Autodesk Inventor part; units mm, degrees
ref_plane "Work Plane1" through (0, -11.5, 75) normal (0, 0, 1) x (1, 0, 0)
ref_plane "YZ Plane" through (0, 0, 0) normal (1, 0, 0) x (0, 1, 0)
ref_plane "XZ Plane" through (0, 0, 0) normal (0, 1, 0) x (-1, 0, 0)
sketch "Sketch1" plane through (0, 0, 0) normal (1, 0, 0) x (0, 1, 0)
  line L0 (0, 0) -> (4.5, 0)
  line L1 (4.5, 0) -> (4.5, 43)
  line L2 (4.5, 43) -> (0, 43)
  line L3 (0, 43) -> (0, 0)
  line L4 (4.5, 43) -> (8.9259, 26.4824)
  line L5 (4.5, 21.5) -> (10.3528, 21.5)
  line L6 (13, 25) -> (10.8577, 25)
  line L7 (25.5, 39.5) -> (30, 39.5)
  line L8 (30, 39.5) -> (30, 3.5)
  line L9 (30, 3.5) -> (25.5, 3.5)
  line L10 (25.5, 3.5) -> (25.5, 39.5)
  line L11 (25.5, 39.5) -> (22.0119, 26.4824)
  line L12 (10.8577, 18) -> (20.0801, 18)
  line L13 (4.5, 0) -> (8.9259, 16.5176)
  line L14 (25.5, 3.5) -> (22.0119, 16.5176)
  line L15 (3, 25) -> (20.0801, 25)
  arc A0 (8.9259, 26.4824) -> (10.8577, 25) centre (10.8577, 27) ccw
  arc A1 (20.0801, 25) -> (22.0119, 26.4824) centre (20.0801, 27) ccw
  arc A2 (22.0119, 16.5176) -> (20.0801, 18) centre (20.0801, 16) ccw
  arc A3 (10.8577, 18) -> (8.9259, 16.5176) centre (10.8577, 16) ccw
  line L16 (-11.5, 16.5176) -> (-11.5, 3.5)
  point P0 (9.6974, 23.6032)
  point P1 (21.6069, 24.9709)
  point P2 (3, 18)
  point P3 (23.25, 18)
  point P4 (9.6974, 19.3968)
  point P5 (21.6069, 18.0291)
  point P6 (23.25, 25)
  dimension "d0" = 43
  dimension "d1" = 4.5
  dimension "d2" = 15
  dimension "d3" = 21.5
  dimension "d4" = 3.5
  dimension "d5" = 4.5
  dimension "d6" = 36
  dimension "d7" = 18
  dimension "d8" = 15
  dimension "d9" = 3.5
  dimension "d10" = 30
  dimension "d11" = 2
  dimension "d12" = 32
revolve "Revolution1" add sketch "Sketch1" angle 360 about axis through (0, -11.5, 16.5176) along (0, 0, -1)
ref_plane "Work Plane1" through (0, -11.5, 75) normal (0, 0, 1) x (1, 0, 0)
sketch "Sketch2" plane through (0, -11.5, 75) normal (0, 0, 1) x (1, 0, 0)
  line L0 (9.2559, 22.3457) -> (12.1824, 29.4109)
  line L1 (22.3457, 9.2559) -> (27.1721, 11.2551)
  line L2 (0, 0) -> (0, 29.4109)
  line L3 (0, 0) -> (29.4109, 0)
  arc A0 (27.3903, 11.3454) -> (11.3454, 27.3903) centre (0, 0) ccw
  line L4 (22.3457, 9.2559) -> (27.1721, 11.2551)
  line L5 (22.3457, 9.2559) -> (27.3903, 11.3454)
  line L6 (22.3457, 9.2559) -> (27.3903, 11.3454)
  arc A1 (22.3457, 9.2559) -> (9.2559, 22.3457) centre (0, 0) ccw
  arc A2 (0, 24.1868) -> (24.1868, 0) centre (0, 0) ccw
  line L7 (11.3454, 27.3903) -> (9.2559, 22.3457)
  line L8 (27.3903, 11.3454) -> (22.3457, 9.2559)
  arc A3 (22.3457, 9.2559) -> (9.2559, 22.3457) centre (0, 0) ccw
  arc A4 (27.3903, 11.3454) -> (11.3454, 27.3903) centre (0, 0) ccw
  line L9 (9.2559, -22.3457) -> (12.1824, -29.4109)
  line L10 (22.3457, -9.2559) -> (27.1721, -11.2551)
  arc A5 (11.3454, -27.3903) -> (27.3903, -11.3454) centre (0, 0) ccw
  line L11 (22.3457, -9.2559) -> (27.1721, -11.2551)
  line L12 (22.3457, -9.2559) -> (27.3903, -11.3454)
  line L13 (22.3457, -9.2559) -> (27.3903, -11.3454)
  arc A6 (9.2559, -22.3457) -> (22.3457, -9.2559) centre (0, 0) ccw
  line L14 (11.3454, -27.3903) -> (9.2559, -22.3457)
  line L15 (27.3903, -11.3454) -> (22.3457, -9.2559)
  arc A7 (9.2559, -22.3457) -> (22.3457, -9.2559) centre (0, 0) ccw
  arc A8 (11.3454, -27.3903) -> (27.3903, -11.3454) centre (0, 0) ccw
  line L16 (0, 0) -> (0, -24.1868)
  line L17 (-9.2559, 22.3457) -> (-12.1824, 29.4109)
  line L18 (-22.3457, 9.2559) -> (-27.1721, 11.2551)
  arc A9 (-11.3454, 27.3903) -> (-27.3903, 11.3454) centre (0, 0) ccw
  line L19 (-22.3457, 9.2559) -> (-27.1721, 11.2551)
  line L20 (-22.3457, 9.2559) -> (-27.3903, 11.3454)
  line L21 (-22.3457, 9.2559) -> (-27.3903, 11.3454)
  arc A10 (-9.2559, 22.3457) -> (-22.3457, 9.2559) centre (0, 0) ccw
  line L22 (-11.3454, 27.3903) -> (-9.2559, 22.3457)
  line L23 (-27.3903, 11.3454) -> (-22.3457, 9.2559)
  arc A11 (-9.2559, 22.3457) -> (-22.3457, 9.2559) centre (0, 0) ccw
  arc A12 (-11.3454, 27.3903) -> (-27.3903, 11.3454) centre (0, 0) ccw
  line L24 (-22.3457, -9.2559) -> (-27.1721, -11.2551)
  line L25 (-22.3457, -9.2559) -> (-27.1721, -11.2551)
  line L26 (-22.3457, -9.2559) -> (-27.3903, -11.3454)
  line L27 (-22.3457, -9.2559) -> (-27.3903, -11.3454)
  line L28 (-27.3903, -11.3454) -> (-22.3457, -9.2559)
  arc A13 (-22.3457, -9.2559) -> (-9.2559, -22.3457) centre (0, 0) ccw
  arc A14 (-22.3457, -9.2559) -> (-9.2559, -22.3457) centre (0, 0) ccw
  arc A15 (-27.3903, -11.3454) -> (-11.3454, -27.3903) centre (0, 0) ccw
  line L29 (-11.3454, -27.3903) -> (-9.2559, -22.3457)
  line L30 (-9.2559, -22.3457) -> (-12.1824, -29.4109)
  arc A16 (-27.3903, -11.3454) -> (-11.3454, -27.3903) centre (0, 0) ccw
  point P0 (0, 11.5)
  point P1 (-29.4109, 0)
  point P2 (-24.1868, 0)
  point P3 (-9.2559, 22.3457)
  point P4 (9.2559, -22.3457)
  point P5 (27.1721, -11.2551)
  point P6 (22.3457, -9.2559)
  point P7 (-22.3457, -9.2559)
  point P8 (-27.1721, -11.2551)
  dimension "d15" = 29.4109
  dimension "d16" = 22.5
  dimension "d17" = 22.5
extrude "Extrusion1" cut sketch "Sketch2" against normal through all contours L0 A0 L5 L1 A1 | A2 L18 L20 A9 L17 | L10 L12 A5 L9 A2 | L29 A15 L26 L24 A2
equation "\"d3\" = 0.5 * d0"
equation "\"d7\" = 0.5 * d6"
properties part number "roller"
Work out the finished part from the listing and answer in its coordinate system (mm). A direction names the side the tool comes from. Round coordinates to 2 decimals unless told otherwise and drop trailing zeros. Loops run counter-clockwise (first coordinate to the right, second up) from the corner with the lowest first, then second, coordinate; pieces in that order, holes last. Notation, with made-up numbers: (-34, 43) -> (-7, 43) arc R24 ccw to (-7, 77) -> close; hole circle Ø3 at (40, 48). An arc over 180 degrees is marked (long way). Write each question's results on one line, items separated by ' | '. Start each with the question number.
1. Section D-D (z = 33.5) is taken. Determine the outline of the cut face in (x, y).
2. Find the intervals of material crossed by probe 1 along X at (y, z) = (-11, 15); probe 2 along X at (y, z) = (-11.5, 12.5); probe 3 along Y at (x, z) = (24, 22.5), in increasing order. Write a range as from..to.
3. For a pull along Y with two mould halves and no side action, classify faces 1 (the face through (-25.252, -44.433, 21.248)), 2 (the face through (-7, -1, 43)), 3 (the face through (-10.315, -36.403, 21.549)) as +Y half, -Y half, draft (parallel to the pull), parting line (faces both ways), or undercut.
4. Given pin 1 Ø1 at (x, z) = (28, 23) entering from -Y; pin 2 Ø3 at (x, z) = (-3.5, 24.5) entering from -Y; pin 3 Ø10 at (y, z) = (-22.5, 23.5) entering from -X, each flat-ended and moving along its own axis, determine where each tip first touches the part or whether it passes through.
5. Section C-C (z = 21) is taken. Determine the outline of the cut face in (x, y).
6. A tool of negligible diameter and unlimited length cuts with its end or side. For faces 4 (the face through (17.008, -28.696, 21.549)), 5 (the face through (-21, -2, 18)), 6 (the face through (-21, -2, 25)), from which of +Z, -Z, +X, -X, +Y, -Y can it reach the whole face along a straight path? Write none if from no direction.
Evaluation:
1) outline: circle Ø83 at (0, -11.5); circle Ø37.09 at (0, -11.5); hole circle Ø70.78 at (0, -11.5); hole circle Ø23 at (0, -11.5)
2) probe 1: x = -41.5..-33.91, -20.01..-11.49, 11.49..20.01, 33.91..41.5 | probe 2: x = -41.5..-34.59, -19.35..-11.5, 11.5..19.35, 34.59..41.5 | probe 3: y = -45.36..-28.91, -21.44..-1.56, 5.91..22.36
3) face 1: parting line | face 2: draft | face 3: undercut
4) pin 1: stops at y = -42.58 | pin 2: stops at y = -52.95 | pin 3: stops at x = -41.06
5) outline: circle Ø83 at (0, -11.5); hole (-27.39, -22.85) arc R29.65 ccw to (-11.35, -38.89) -> (-9.26, -33.85) arc R24.19 cw to (-22.35, -20.76) -> (-27.17, -22.76) -> close; hole (-27.39, -0.15) -> (-27.17, -0.24) -> (-22.35, -2.24) arc R24.19 cw to (-9.26, 10.85) -> (-11.35, 15.89) arc R29.65 ccw to start; hole circle Ø23 at (0, -11.5); hole (9.26, -33.85) -> (11.35, -38.89) arc R29.65 ccw to (27.39, -22.85) -> (27.17, -22.76) -> (22.35, -20.76) arc R24.19 cw to start; hole (9.26, 10.85) arc R24.19 cw to (22.35, -2.24) -> (27.17, -0.24) -> (27.39, -0.15) arc R29.65 ccw to (11.35, 15.89) -> close
6) face 4: +Z, -Z | face 5: -Z | face 6: +Z
